```python
from build123d import *

# Parameters (mm, degrees)
F0_R     = 7.5
F1_DEPTH = 9
F2_R     = 7.5
F3_DEPTH = 21


with BuildPart() as f1:
    # F0 (on Top) → F1 (new body)
    with BuildSketch(Plane.XY):
        with BuildLine():
            Line((-0.11538, 0), (17.88462, 0))
            Line((17.88462, 0), (17.88462, 30))
            Line((17.88462, 30), (-0.11538, 30))
            ThreePointArc((-0.11538, 30), (-15.11538, 15), (-0.11538, 0))
        make_face()
        with Locations((-0.11538, 15)):
            Circle(F0_R, mode=Mode.SUBTRACT)
        Polygon((17.88462, 30), (17.88462, 0), (49.807702, 0), (59.88462, 9), (59.88462, 21), (49.230773, 30), align=None)
    extrude(amount=F1_DEPTH)

    # F2 (on face) → F3 (join)
    with BuildSketch(Plane.XY.offset(9)):
        with BuildLine():
            Line((17.88462, 0), (17.88462, 30))
            Line((17.88462, 30), (-0.11538, 30))
            ThreePointArc((-0.11538, 30), (-15.11538, 15), (-0.11538, 0))
            Line((-0.11538, 0), (17.88462, 0))
        make_face()
        with Locations((-0.11538, 15)):
            Circle(F2_R, mode=Mode.SUBTRACT)
    extrude(amount=F3_DEPTH)


solid = f1.part
```
Model file for the job. Use its own axes, mm. A direction names the side the tool comes from. Give positions to 0.01 mm unless a question says otherwise; leave off trailing zeros. Loops run counter-clockwise (first coordinate to the right, second up) from the corner with the lowest first, then second, coordinate; pieces in that order, holes last. Notation, with made-up numbers: M 14.25,21.25 L 70.25,21.25 A5 cw 70.25,26.25 Z; hole C 77,-37.5 d8. An arc over 180 degrees is marked long. Use one line per item in the form item = value.
Item 1: Which spindle directions (+Z, -Z, +X, -X, +Y, -Y) get a long thin tool onto all of the face, cutting with end or side? Do faces 1 (the flat face through (17.885, 15, 19)), 2 (the flat face through (54.78, 4.44, 4.44)). Say none if no direction does.
Filled in:
face_1 = +Z, +X, +Y, -Y
face_2 = +Z, -Z, +X, -Y
Item 2: Flat gauge pins, fed straight in: pin 1 Ø4 at (y, z) = (21, 23.5) entering from -X; pin 2 Ø8 at (x, y) = (51, 21) entering from +Z; pin 3 Ø17 at (y, z) = (15.5, 18.5) entering from +X. Where does each tip first touch, or does it go through?
Filled in:
pin_1 = -14.57
pin_2 = 9
pin_3 = 17.88
Item 3: Slice it at B-B on z = 22.75. List the corners of the cut face in (x, y), and give its area (3 significant figures).
Filled in:
outline = M -0.12,0 L 17.88,0 L 17.88,30 L -0.12,30 A15 ccw Z; hole C -0.12,15 d15
area = 717 mm^2
Item 4: Slice it at D-D on z = 3.75. List the corners of the cut face in (x, y), and give its area (3 significant figures).
Filled in:
outline = M -0.12,0 L 49.81,0 L 59.88,9 L 59.88,21 L 49.23,30 L -0.12,30 A15 ccw Z; hole C -0.12,15 d15
area = 1,880 mm^2
Item 5: Two-plate mould, pull along X, no slides. Class faces 3 (the flat face through (19, 0, 8)), 4 (the cylindrical face through (-15.11, 15.33, 14.79)), 5 (the cylindrical face through (7.04, 17.25, 14.79)), 6 (the flat face through (54.63, 25.44, 4.44)): released by +X, released by -X, zero draft, split by the parting line, or undercut.
Filled in:
face_3 = zero draft
face_4 = released by -X
face_5 = undercut
face_6 = released by +X
Item 6: Drill centre lines: L1, parallel to Z at x = 33, y = 25.75; L2, parallel to X at y = 20, z = 13; L3, parallel to Y at x = -3, z = 9.25. Where is each one in solid material? Low to high.
Filled in:
L1 = 0 to 9
L2 = -14.26 to -5.71, 5.47 to 17.88
L3 = 0.28 to 8.08, 21.92 to 29.72
Item 7: Slice it at A-A on y = 15. List the corners of the cut face in (x, z), and give its area (3 significant figures).
Filled in:
outline = M -15.12,0 L -7.62,0 L -7.62,30 L -15.12,30 Z; M 7.38,0 L 59.88,0 L 59.88,9 L 17.88,9 L 17.88,30 L 7.38,30 Z
area = 918 mm^2
Item 8: Slice it at C-C on x = 1.5. List the corners of the cut face in (y, z).
Filled in:
outline = M 0,0 L 7.68,0 L 7.68,30 L 0,30 Z; M 22.32,0 L 30,0 L 30,30 L 22.32,30 Z
